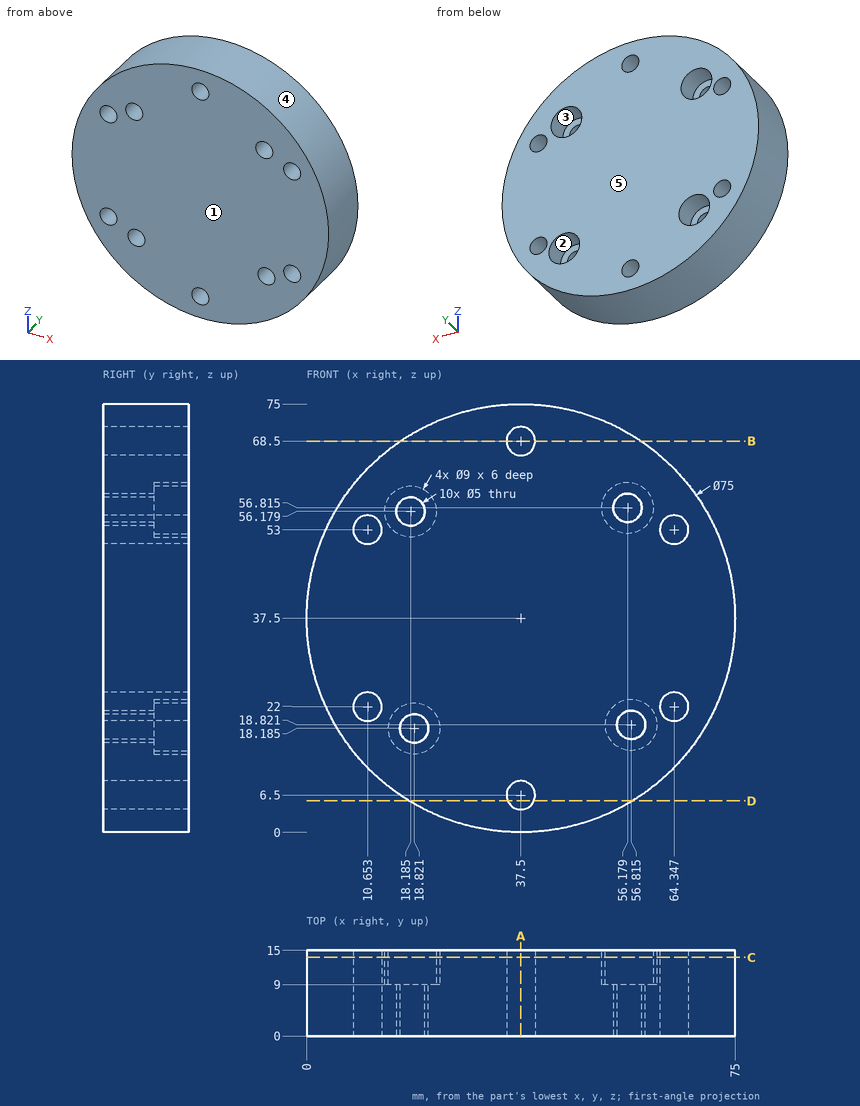
Job drawing, mm, ordinate dimensions from the low corner. One solid piece. A direction names the side the tool comes from. Coordinates: 2 decimals unless noted, no trailing zeros. Order: outer loops, then holes, each group sorted by start corner. A loop starts at its lowest first (then second) coordinate and runs counter-clockwise, first axis right, second up. Notation, with made-up numbers: (-15.75, 38) -> (-8.75, 38) arc R30 ccw to (-8.75, 75) -> close; hole circle Ø8 at (14, 6.5). An arc over 180 degrees is marked (long way). Return JSON: item names as keys, results as strings. Group by question number.
Item 1: Saw through at A-A on x = 37.5. Write the cut outline in (y, z), then the cut area to 3 significant figures.
Item 2: Tool access for the marked faces 1 and 2: list every direction of +Z, -Z, +X, -X, +Y, -Y with a clear straight run to the whole face (end or side of a thin tool).
Item 3: Saw through at B-B on z = 68.5. Write the cut outline in (x, y).
Item 4: Saw through at C-C on y = 13.75. State how many separate pieces and enclosed holes the cut face has, then the cut area to 3 significant figures.
Item 5: Pull direction X, two halves, no side cores. Call the marked faces 3, 4 and 5: pulls with the +X half, pulls with the -X half, needs draft (parallel to the pull), parting line crosses it, or undercut.
Item 6: Wall check: line 1 along X through (y, z) = (4, 54) (1 decimal); line 2 along Z through (x, y) = (11, 4.75) (1 decimal); line 3 along Z through (x, y) = (66, 4.25) (1 decimal). Give the ranges that are in metal, low to high. Write a range as [from, to].
Item 7: Flat gauge pins, fed straight in: P1, Ø4, axis at x = 46, y = 10.5, coming from the +Z side; P2, Ø6, axis at x = 56.82, z = 18.82, coming from the +Y side; P3, Ø2, axis at y = 1.5, z = 62, coming from the -X side; P4, Ø3, axis at x = 10.65, z = 53, coming from the +Y side. Where does each tip first touch, or does it go through?
Item 8: Saw through at D-D on z = 5.5. Write the cut outline in (x, y).
Values found:
{
 "1": {"outline": "(0, 0) -> (15, 0) -> (15, 4) -> (0, 4) -> close; (0, 9) -> (15, 9) -> (15, 66) -> (0, 66) -> close; (0, 71) -> (15, 71) -> (15, 75) -> (0, 75) -> close", "area": "975 mm2"},
 "2": {"face 1": "+Z, -Z, +X, -X, -Y", "face 2": "+Y"},
 "3": {"outline": "(16.4, 0) -> (35, 0) -> (35, 15) -> (16.4, 15) -> close; (40, 0) -> (58.6, 0) -> (58.6, 15) -> (40, 15) -> close"},
 "4": {"separate pieces": "1", "enclosed holes": "10", "area": "4,050 mm2"},
 "5": {"face 3": "undercut", "face 4": "parting line crosses it", "face 5": "needs draft"},
 "6": {"line 1": "x = [3.8, 8.4], [12.9, 17], [19.4, 62.1], [66.6, 71.2]", "line 2": "z = [11, 19.5], [24.5, 50.5], [55.5, 64]", "line 3": "z = [13.1, 20.1], [23.9, 51.1], [54.9, 61.9]"},
 "7": {"P1": "stops at z = 74.43", "P2": "stops at y = 9", "P3": "stops at x = 8.28", "P4": "passes through"},
 "8": {"outline": "(17.95, 0) -> (35.21, 0) -> (35.21, 15) -> (17.95, 15) -> close; (39.79, 0) -> (57.05, 0) -> (57.05, 15) -> (39.79, 15) -> close"}
}
